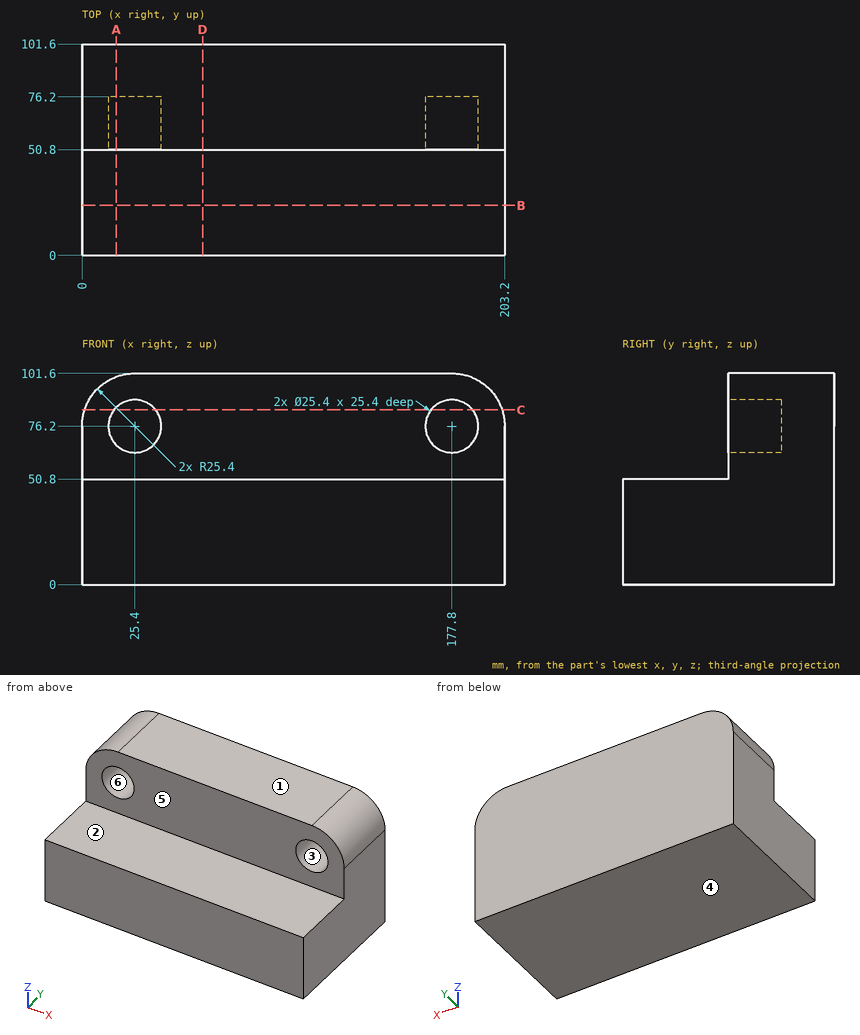
Drawing for the job (mm, zero at the part's lowest x, y, z). A direction names the side the tool comes from. Round coordinates to 2 decimals unless told otherwise and drop trailing zeros. Order: outer loops, then holes, each group sorted by start corner. A loop starts at its lowest first (then second) coordinate and runs counter-clockwise, first axis right, second up.
Item 1: Pin check, flat tips, straight feed: pin 1 (1.5 mm diameter, centred on y = 48.5, z = 57.5, fed in from -X); pin 2 (6 mm diameter, centred on x = 67, y = 26, fed in from +Z); pin 3 (7.5 mm diameter, centred on x = 23, z = 71, fed in from -Y); pin 4 (15 mm diameter, centred on x = 72.5, z = 71, fed in from -Y). Stop position of each tip, or through.
Item 2: Probe line 1 along X through (y, z) = (56, 76); line 2 along Z through (x, y) = (26, 55); line 3 along Y through (x, z) = (158.5, 75.5). List the from-to ranges inside material, lowest first.
Item 3: Tool access for the marked faces 1 and 2: list every direction of +Z, -Z, +X, -X, +Y, -Y with a clear straight run to the whole face (end or side of a thin tool).
Item 4: Saw through at B-B on y = 24. Write the cut outline in (x, z).
Item 5: Mould opens along Z. For the marked faces 3, 4, 5 and 6 say: pulls with the +Z half, pulls with the -Z half, needs draft (parallel to the pull), parting line crosses it, or undercut.
Item 6: Saw through at A-A on x = 16.5. Write the cut outline in (y, z), then the cut area to 3 significant figures.
Item 7: Saw through at C-C on z = 84. Write the cut outline in (x, y), then the cut area to 3 significant figures.
Item 8: Saw through at D-D on x = 58. Write the cut outline in (y, z), then the cut area to 3 significant figures.
Reported:
1. pin 1: passes through
1. pin 2: stops at z = 50.8
1. pin 3: stops at y = 76.2
1. pin 4: stops at y = 50.8
2. line 1: x = 0 to 12.7, 38.1 to 165.1, 190.5 to 203.2
2. line 2: z = 0 to 63.51, 88.89 to 101.6
2. line 3: y = 50.8 to 101.6
3. face 1: +Z, +X, -X, +Y, -Y
3. face 2: +Z, +X, -X, -Y
4. outline: (0, 0) - (203.2, 0) - (203.2, 50.8) - (0, 50.8) - close
5. face 3: undercut
5. face 4: pulls with the -Z half
5. face 5: needs draft
5. face 6: undercut
6. outline: (0, 0) - (101.6, 0) - (101.6, 99.99) - (50.8, 99.99) - (50.8, 85.26) - (76.2, 85.26) - (76.2, 67.14) - (50.8, 67.14) - (50.8, 50.8) - (0, 50.8) - close
6. area: 7,200 mm2
7. outline: (1.23, 50.8) - (15.38, 50.8) - (15.38, 76.2) - (35.42, 76.2) - (35.42, 50.8) - (167.78, 50.8) - (167.78, 76.2) - (187.82, 76.2) - (187.82, 50.8) - (201.97, 50.8) - (201.97, 101.6) - (1.23, 101.6) - close
7. area: 9,180 mm2
8. outline: (0, 0) - (101.6, 0) - (101.6, 101.6) - (50.8, 101.6) - (50.8, 50.8) - (0, 50.8) - close
8. area: 7,740 mm2
